Read the model definition and answer for the solid it produces. Units are mm, in the model's axes. Face numbers are marked on the shaded views. A direction names the side the tool comes from. Coordinates: 2 decimals unless noted, no trailing zeros. Order: outer loops, then holes, each group sorted by start corner. A loop starts at its lowest first (then second) coordinate and runs counter-clockwise, first axis right, second up.
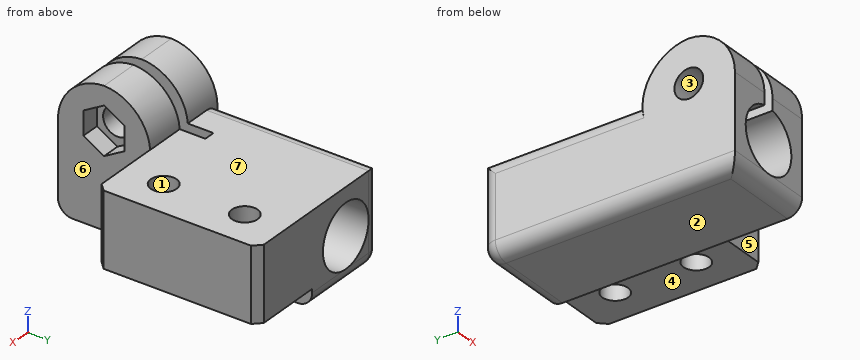
```python
from build123d import *

# Parameters (mm, degrees)
F0_W         = 25
F0_H         = 44
F0_H_2       = 25
F1_DEPTH     = 25
F0_W_2       = 20
F0_R         = 3.5
F2_DEPTH     = 25
F3_R         = 8.5
F4_DEPTH     = 69.001
F5_W         = 11
F5_H         = 25.0466239899
F6_DEPTH     = 12
F5_W_2       = 3
F5_H_2       = 6.9533760101
F7_DEPTH     = 4.1343997347
F9_T1_DEPTH  = 76
F9_T3_DEPTH  = 76
F9_T5_DEPTH  = 75.8074069841
F9_T7_DEPTH  = 75.8074069841
F10_DEPTH    = 5
F8_R         = 3.9
F11_DEPTH    = 25.001
F12_DEPTH    = 25.001
F13_DEPTH    = 5
F14_R        = 3.99999
F15_T1_DEPTH = 30.2867319519


# Not quite as in the source:
# - a fillet or chamfer that OpenCascade refuses, or shapes differently, is made with other operations: its cross-section is extruded or revolved along the edge and cut away or added
# - a fillet or chamfer is up to 0.001 mm smaller than in the source, because OpenCascade refuses the exact size
# - a feature names something its author has since deleted; it is built from what else it names


with BuildPart() as f1:
    # F0 (on Top) → F1 (new body)
    with BuildSketch(Plane.XY):
        Rectangle(F0_W, F0_H)
        with Locations((0, -34.5)):
            Rectangle(F0_W, F0_H_2)
    extrude(amount=F1_DEPTH)

    # F0 (on Top) → F2 (join)
    with BuildSketch(Plane.XY):
        with Locations((22.5, 0)):
            Rectangle(F0_W_2, F0_H)
        with Locations((22.5, -11)):
            Circle(F0_R, mode=Mode.SUBTRACT)
        with Locations((22.5, 11)):
            Circle(F0_R, mode=Mode.SUBTRACT)
    extrude(amount=F2_DEPTH)

    # F3 (on face) → F4 (cut, through all)
    with BuildSketch(Plane.XZ.offset(47)):
        with Locations((0, 12.5)):
            Circle(F3_R)
    extrude(amount=-F4_DEPTH, mode=Mode.SUBTRACT)

    # F5 (on face) → F6 (join)
    with BuildSketch(Plane.XY.offset(25)):
        with Locations((-7, -34.476688005)):
            Rectangle(F5_W, F5_H)
        Polygon((12.5, -22), (12.5, -21.9533760101), (1.5, -21.9533760101), (1.5, -47), (12.5, -47), align=None)
    extrude(amount=F6_DEPTH)

    # F5 (on face) → F7 (cut, through all)
    with BuildSketch(Plane.XY.offset(25)):
        with Locations((0, -34.476688005)):
            Rectangle(F5_W_2, F5_H)
        with Locations((0, -18.476688005)):
            Rectangle(F5_W_2, F5_H_2)
    extrude(amount=-F7_DEPTH, mode=Mode.SUBTRACT)

    # F9: fillet of radius 13 on 4 edges, made by hand

    # F9_s2 → F9_t1 (cut)
    with BuildSketch(Plane.YZ.offset(-45)):
        with BuildLine():
            ThreePointArc((-34, 37), (-43.1923881554, 33.1923881554), (-47, 24))
            Line((-47, 24), (-47, 37))
            Line((-47, 37), (-34, 37))
        make_face()
    extrude(amount=F9_T1_DEPTH, mode=Mode.SUBTRACT)

    # F9_s4 → F9_t3 (cut)
    with BuildSketch(Plane.YZ.offset(-31)):
        with BuildLine():
            ThreePointArc((-34, 37), (-43.1923881554, 33.1923881554), (-47, 24))
            Line((-47, 24), (-47, 37))
            Line((-47, 37), (-34, 37))
        make_face()
    extrude(amount=F9_T3_DEPTH, mode=Mode.SUBTRACT)

    # F9_s6 → F9_t5 (cut)
    with BuildSketch(Plane.YZ.offset(-30.903703492)):
        with BuildLine():
            ThreePointArc((-34.9148574069, 37), (-26.0830965405, 33.5393920142), (-21.9533760101, 25))
            Line((-21.9533760101, 25), (-21.9533760101, 37))
            Line((-21.9533760101, 37), (-34.9148574069, 37))
        make_face()
    extrude(amount=F9_T5_DEPTH, mode=Mode.SUBTRACT)

    # F9_s8 → F9_t7 (cut)
    with BuildSketch(Plane.YZ.offset(-44.903703492)):
        with BuildLine():
            ThreePointArc((-21.9533760101, 25), (-26.0830965405, 33.5393920142), (-34.9148574069, 37))
            Line((-34.9148574069, 37), (-21.9533760101, 37))
            Line((-21.9533760101, 37), (-21.9533760101, 25))
        make_face()
    extrude(amount=F9_T7_DEPTH, mode=Mode.SUBTRACT)

    # F0 (on Top) → F10 (cut)
    with BuildSketch(Plane.XY):
        with Locations((22.5, 0)):
            Rectangle(F0_W_2, F0_H)
        with Locations((22.5, -11)):
            Circle(F0_R, mode=Mode.SUBTRACT)
        with Locations((22.5, 11)):
            Circle(F0_R, mode=Mode.SUBTRACT)
    extrude(amount=F10_DEPTH, mode=Mode.SUBTRACT)

    # F8 (on face) → F11 (cut, through all)
    with BuildSketch(Plane.YZ.offset(12.5)):
        with Locations((-34.476688005, 25.4739885092)):
            Circle(F8_R)
    extrude(amount=-F11_DEPTH, mode=Mode.SUBTRACT)

    # F8 (on face) → F12 (cut, through all)
    with BuildSketch(Plane.YZ.offset(12.5)):
        with Locations((-34.476688005, 25.4739885092)):
            Circle(F8_R)
    extrude(amount=-F12_DEPTH, mode=Mode.SUBTRACT)

    # F8 (on face) → F13 (cut)
    with BuildSketch(Plane.YZ.offset(12.5)):
        Polygon((-40.076688005, 28.7071500166), (-40.076688005, 22.2408270017), (-34.476688005, 19.0076654943), (-28.876688005, 22.2408270017), (-28.876688005, 28.7071500166), (-34.476688005, 31.9403115241), align=None)
        with Locations((-34.476688005, 25.4739885092)):
            Circle(F8_R, mode=Mode.SUBTRACT)
    extrude(amount=-F13_DEPTH, mode=Mode.SUBTRACT)

    # F14 (radius 4 in the source; OpenCascade refuses exactly that, so slightly less here)
    f14_edges = [f1.edges().sort_by_distance(p)[0] for p in [
        (-12.5, -12.5, 0),
        (0, -47, 0),
        (-12.5, 0.023312, 25),
        (0, 22, 0),
        (-12.5, 22, 12.5),
    ]]
    fillet(f14_edges, radius=F14_R)

    # F15: chamfer of 2 on 2 edges, made by hand

    # F15_s2 → F15_t1 (cut)
    with BuildSketch(Plane.XY.offset(-0.1433659759)):
        Polygon((30.5, 22), (32.5, 20), (32.5, 22), align=None)
        Polygon((32.5, -20), (30.5, -22), (32.5, -22), align=None)
    extrude(amount=F15_T1_DEPTH, mode=Mode.SUBTRACT)


solid = f1.part
```
1) Straight lines are drawn through the part: line 1 (X direction, y = -39, z = 35.5); line 2 (Y direction, x = 21.5, z = 20); line 3 (Y direction, x = 20, z = 17). For each, find the intervals that lie inside material, in ascending order.
A:
line 1: x = -12.5 to -1.5, 1.5 to 12.5
line 2: y = -22 to -14.35, -7.65 to 7.65, 14.35 to 22
line 3: y = -22 to -13.45, -8.55 to 8.55, 13.45 to 22
2) A cutting plane is placed at B-B, the plane y = 11. Determine the outline of the cut face in (x, z), and give its area (3 significant figures).
A:
outline: (-12.5, 4) arc R4 ccw to (-8.5, 0) - (12.5, 0) - (12.5, 5) - (19, 5) - (19, 25) - (-8.5, 25) arc R4 ccw to (-12.5, 21) - close; (26, 5) - (32.5, 5) - (32.5, 25) - (26, 25) - close; hole circle Ø17 at (0, 12.5)
area: 651 mm2
3) A cutting plane is placed at A-A, the plane z = 12.5. State how many separate pieces and enclosed holes the cut face has, and give its area (3 significant figures).
A:
separate pieces: 2
enclosed holes: 2
area: 1,350 mm2
4) A cutting plane is placed at C-C, the plane x = 22.5. Determine the outline of the cut face in (y, z).
A:
outline: (-22, 5) - (-14.5, 5) - (-14.5, 25) - (-22, 25) - close; (-7.5, 5) - (7.5, 5) - (7.5, 25) - (-7.5, 25) - close; (14.5, 5) - (22, 5) - (22, 25) - (14.5, 25) - close
5) Determine the mould class of the marked faces 1, 2 and 3 for opening direction Z: pulls with the +Z half, pulls with the -Z half, needs draft (parallel to the pull), parting line crosses it, or undercut.
A:
face 1: needs draft
face 2: pulls with the -Z half
face 3: undercut
6) A cutting plane is placed at D-D, the plane x = -2.5. Determine the outline of the cut face in (y, z).
A:
outline: (-47, 4) arc R4 ccw to (-43, 0) - (18, 0) arc R4 ccw to (22, 4) - (22, 4.38) - (-47, 4.38) - close; (-47, 20.62) - (22, 20.62) - (22, 25) - (-21.95, 25) arc R13 ccw to (-34.46, 36.99) arc R13 ccw to (-47, 24) - close; hole circle Ø7.8 at (-34.48, 25.47)
7) Flat-ended cylindrical pins translate along their axes: pin 1 Ø6.5 at (x, y) = (22.5, 11) entering from -Z; pin 2 Ø9 at (y, z) = (-34.48, 25.47) entering from +X; pin 3 Ø8 at (x, y) = (22.5, -11) entering from +Z; pin 4 Ø5 at (x, z) = (15.5, 19.5) entering from -Y. Find the tip coordinate at first contact, or state that the pin passes through.
A:
pin 1: passes through
pin 2: stops at x = 7.5
pin 3: stops at z = 25
pin 4: stops at y = -22
8) Which of the six approach directions +Z, -Z, +X, -X, +Y, -Y give full straight-line access (tool end or side, diameter ignored) to the marked faces 4, 5, 6 and 7?
A:
face 4: -Z, +X, +Y, -Y
face 5: +Z, -Z, +X, -Y
face 6: -Z, +X, -Y
face 7: +Z, +X, -X, +Y
